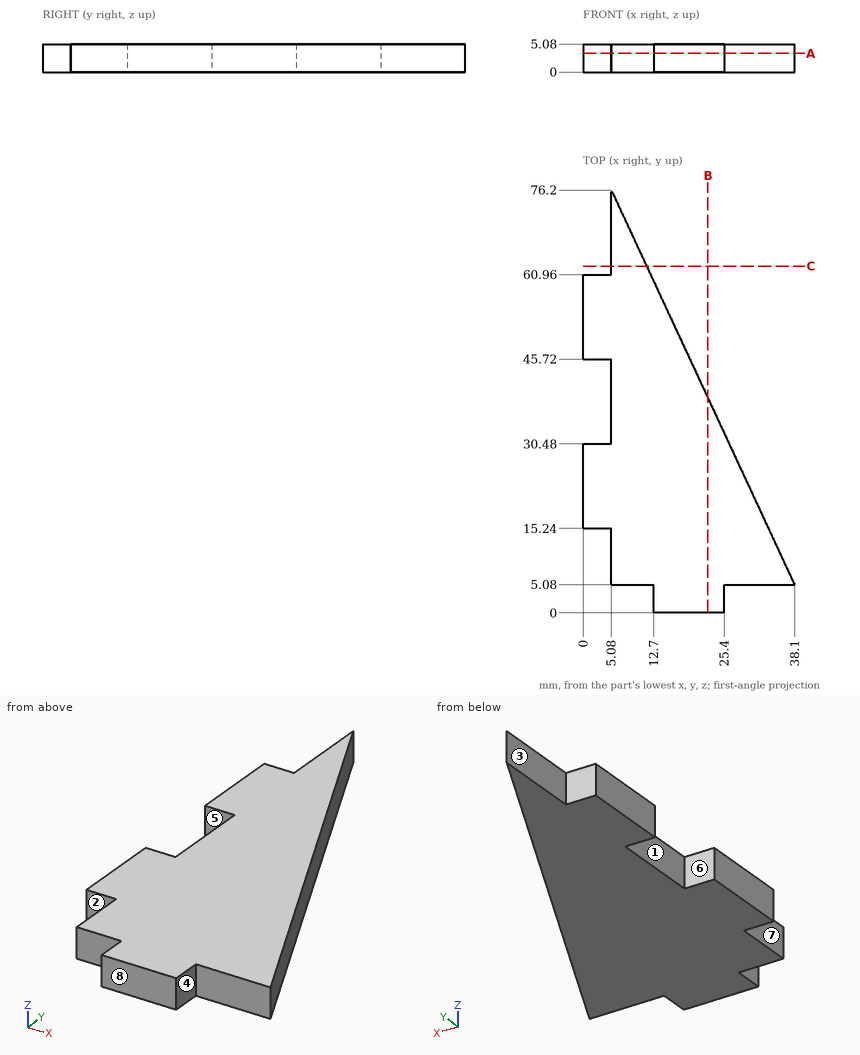
Here's the drawing with two shaded views (mm, measured from the low corner). I have some questions. A direction names the side the tool comes from. Coordinates: 2 decimals unless noted, no trailing zeros. Order: outer loops, then holes, each group sorted by start corner. A loop starts at its lowest first (then second) coordinate and runs counter-clockwise, first axis right, second up. Notation, with made-up numbers: (79.5, 0) -> (124.5, 0) arc R22 ccw to (124.5, 32) -> close; hole circle Ø4 at (-40, -40). An arc over 180 degrees is marked (long way). One line per question, with ' | ' between items.
Q1. Imagine slicing it at A-A on z = 3.4. Please give me the cut outline in (x, y), and give its area (3 significant figures).
Return value:
outline: (0, 15.24) -> (5.08, 15.24) -> (5.08, 5.08) -> (12.7, 5.08) -> (12.7, 0) -> (25.4, 0) -> (25.4, 5.08) -> (38.1, 5.08) -> (5.08, 76.2) -> (5.08, 60.96) -> (0, 60.96) -> (0, 45.72) -> (5.08, 45.72) -> (5.08, 30.48) -> (0, 30.48) -> close | area: 1,390 mm²
Q2. I'm going to push flat-ended pins straight in: P1, Ø6, axis at x = 18.5, y = 46, coming from the -Z side; P2, Ø1.5, axis at x = 2, z = 1.5, coming from the -Y side; P3, Ø1.5, axis at y = 35, z = 1.5, coming from the -X side; P4, Ø1.5, axis at x = 2, z = 3.5, coming from the +Y side. Where does each tip first touch, or does it pass through?
Return value:
P1: z = 0 | P2: y = 15.24 | P3: x = 5.08 | P4: y = 60.96
Q3. On a 3-axis mill with a long thin cutter (end or side, diameter ignored), from which of +Z, -Z, +X, -X, +Y, -Y can I reach the whole of each face in a straight line? I mean the marked faces 1, 2, 3 and 4. Say none if no direction works.
Return value:
face 1: +Z, -Z, -X | face 2: +Z, -Z, -X, -Y | face 3: +Z, -Z, -X, +Y | face 4: +Z, -Z, +X, -Y
Q4. Imagine slicing it at C-C on y = 62.5. Please give me the cut outline in (x, z), and give its area (3 significant figures).
Return value:
outline: (5.08, 0) -> (11.44, 0) -> (11.44, 5.08) -> (5.08, 5.08) -> close | area: 32.3 mm²
Q5. Imagine slicing it at B-B on x = 22.5. Please give me the cut outline in (y, z).
Return value:
outline: (0, 0) -> (38.68, 0) -> (38.68, 5.08) -> (0, 5.08) -> close
Q6. If I drill on L1, parallel to Y at x = 25, z = 1.8; L2, parallel to X at y = 62.5, z = 2.6; L3, parallel to Y at x = 27, z = 3.8, over which ranges is the centre line in solid material (lowest first)?
Return value:
L1: 0 to 33.3 | L2: 5.08 to 11.44 | L3: 5.08 to 28.99
Q7. Thinking about a two-plate mould opening in Y: for the marked faces 5, 6, 7 and 8, which applies, pulls with the +Y half, pulls with the -Y half, needs draft (parallel to the pull), parting line crosses it, or undercut?
Return value:
face 5: undercut | face 6: undercut | face 7: needs draft | face 8: pulls with the -Y half
